```python
from build123d import *

# Parameters (mm, degrees)
SKETCH1_R           = 12.5
BOSS_EXTRUDE1_DEPTH = 133
SKETCH2_R           = 10
BOSS_EXTRUDE2_DEPTH = 20
FILLET1_R           = 0.5


# Read off the part's stored shape, not the designer's step: M12 Machine Threads Stud1
with BuildPart() as part:
    # Sketch1 → Boss-Extrude1 (new body)
    with BuildSketch(Plane(origin=(0, 0, 0), x_dir=(1, 0, 0), z_dir=(0, 1, 0))):
        with Locations(Location((0, 0, 0), (0, 0, 270))):
            Circle(SKETCH1_R)
    extrude(amount=BOSS_EXTRUDE1_DEPTH)

    # Sketch2 → Boss-Extrude2 (add)
    with BuildSketch(Plane.XZ):
        with Locations(Location((0, 0, 0), (0, 0, 270))):
            Circle(SKETCH2_R)
    extrude(amount=BOSS_EXTRUDE2_DEPTH)

    # M12 Machine Threads Stud1 outline → M12 Machine Threads Stud1 (revolve, cut)
    with BuildSketch(Plane.XY):
        Polygon((10, 0), (6, 0), (6, -19.036), (5.036, -20), (10, -20), align=None)
    revolve(axis=Axis((0, 0, 0), (0, 1, 0)), mode=Mode.SUBTRACT)

    # Fillet1
    fillet1_edges = [part.edges().sort_by_distance(p)[0] for p in [
        (0, 133, -12.5),
    ]]
    fillet(fillet1_edges, radius=FILLET1_R)


solid = part.part
```
For this review, take the finished solid that the model builds, in its own axes (mm). A direction names the side the tool comes from. Round coordinates to 2 decimals unless told otherwise and drop trailing zeros. Write each loop counter-clockwise with the first axis right and the second up, starting at its lowest first coordinate (ties: lowest second). Pieces come first, ordered by that corner, then holes. Notation, with made-up numbers: (-20, 57.5) -> (-16, 57.5) arc R37 cw to (-16, 94.5) -> close; hole circle Ø8 at (32, 76.5). An arc over 180 degrees is marked (long way). One line per question, with ' | ' between items. Start each with the question number.
1) Add section B-B (x = 0). Write out the cut boundary in (y, z), and give its area (3 significant figures).
2) Add section A-A (z = 0). Write out the cut boundary in (x, y), and give its area (3 significant figures).
3) For pin 1 Ø1.5 at (x, y) = (6.5, 85) entering from -Z; pin 2 Ø7.5 at (x, z) = (3, 5.5) entering from -Y; pin 3 Ø6 at (x, y) = (-8.5, 117.5) entering from -Z (3 decimals); pin 4 Ø1.5 at (x, z) = (-6.5, 4.5) entering from -Y, all flat-tipped, find the tip position at first contact; note any pin that passes through.
4) Wall thickness on line 1 along Y through (x, z) = (-10, 1.5); line 2 along Z through (x, y) = (0.25, 15); line 3 along Z through (x, y) = (3.5, 64.5): over which ranges is each line inside the solid? List them lowest first.
5) Machinability: for faces 1 (the flat face through (0, -20, 0)), 2 (the flat face through (3, 0, 5.4)), which of the approach directions +Z, -Z, +X, -X, +Y, -Y give a long, thin tool a straight path to every point of the face, cutting with its end or side? Answer none if there is none.
Reported:
1) outline: (-20, -5.04) -> (-19.04, -6) -> (0, -6) -> (0, -12.5) -> (132.5, -12.5) arc R0.5 ccw to (133, -12) -> (133, 12) arc R0.5 ccw to (132.5, 12.5) -> (0, 12.5) -> (0, 6) -> (-19.04, 6) -> (-20, 5.04) -> close | area: 3,560 mm²
2) outline: (-12.5, 0) -> (-6, 0) -> (-6, -19.04) -> (-5.04, -20) -> (5.04, -20) -> (6, -19.04) -> (6, 0) -> (12.5, 0) -> (12.5, 132.5) arc R0.5 ccw to (12, 133) -> (-12, 133) arc R0.5 ccw to (-12.5, 132.5) -> close | area: 3,560 mm²
3) pin 1: stops at z = -11.1 | pin 2: stops at y = -20 | pin 3: stops at z = -11.225 | pin 4: stops at y = 0
4) line 1: y = 0 to 133 | line 2: z = -12.5 to 12.5 | line 3: z = -12 to 12
5) face 1: +Z, -Z, +X, -X, -Y | face 2: -Y
